CAD build for the part. Positions are in the model's coordinates, mm. A direction names the side the tool comes from. Round coordinates to 2 decimals unless told otherwise and drop trailing zeros. Loops run counter-clockwise (first coordinate to the right, second up) from the corner with the lowest first, then second, coordinate; pieces in that order, holes last. Notation, with made-up numbers: (11, -39) - (64, -39) arc R17 cw to (64, -35) - close; hole circle Ø3 at (19, 0). An arc over 180 degrees is marked (long way). Use one line per item in the form item = value.
Autodesk Inventor part; units mm, degrees
ref_plane "YZ Plane" through (0, 0, 0) normal (1, 0, 0) x (0, 1, 0)
ref_plane "XZ Plane" through (0, 0, 0) normal (0, 1, 0) x (-1, 0, 0)
ref_plane "XY Plane" through (0, 0, 0) normal (0, 0, 1) x (1, 0, 0)
sketch "Sketch1" plane through (0, 0, 0) normal (0, 0, 1) x (1, 0, 0)
  circle A0 centre (0, 0) radius 2.5
  dimension "d0" = 5
extrude "Extrusion1" add sketch "Sketch1" along normal blind 10
sketch "Sketch2" plane through (0, 0, 10) normal (0, 0, 1) x (1, 0, 0)
  circle A0 centre (0, 0) radius 3.5
  dimension "d3" = 7
extrude "Extrusion2" add sketch "Sketch2" along normal blind 4.5
sketch "Sketch3" plane through (0, 0, 14.5) normal (0, 0, 1) x (1, 0, 0)
  line L0 (-1.25, 1.55) -> (1.25, 1.55)
  line L1 (1.25, 1.55) -> (1.25, -1.55)
  line L2 (1.25, -1.55) -> (-1.25, -1.55)
  line L3 (-1.25, -1.55) -> (-1.25, 1.55)
  point P0 (0, 0)
  point P1 (-1.25, 0)
  point P2 (0, 1.55)
  dimension "d6" = 2.5
  dimension "d7" = 3.1
extrude "Extrusion3" cut sketch "Sketch3" against normal blind 4
sketch "Sketch4" plane through (0, 0, 0) normal (0, 0, -1) x (-1, 0, 0)
  circle A0 centre (0, 0) radius 0.5
  line L0 (2.5, -0.1) -> (-2.5, -0.1)
  line L1 (-2.5, -0.1) -> (-2.5, 0.1)
  line L2 (-2.5, 0.1) -> (2.5, 0.1)
  line L3 (2.5, 0.1) -> (2.5, -0.1)
  point P0 (0, -0.1)
  point P1 (2.5, 0)
  point P2 (-0.4899, 0.1)
  point P3 (-0.4899, -0.1)
  point P4 (0.4899, -0.1)
  point P5 (0.4899, 0.1)
  dimension "d10" = 1
  dimension "d11" = 5
  dimension "d12" = 0.2
extrude "Extrusion4" cut sketch "Sketch4" against normal blind 8
properties part number "Magnethalter"
1) Tool access for faces 4 (the flat face through (0, 1, 0)), 5 (the flat face through (1, -0.1, 4)), 6 (the flat face through (2, 0, 14.5)), 7 (the flat face through (1.25, 0, 13)), 8 (the flat face through (0, 0, 8)): list every direction of +Z, -Z, +X, -X, +Y, -Y with a clear straight run to the whole face (end or side of a thin tool).
Report:
face_4 = -Z, +X, -X, +Y, -Y
face_5 = -Z, +X, -X
face_6 = +Z, +X, -X, +Y, -Y
face_7 = +Z
face_8 = -Z
2) Slice it at A-A (x = 0). Write the cut outline in (y, z).
Report:
outline = (-3.5, 10) - (-2.5, 10) - (-2.5, 0) - (-0.5, 0) - (-0.5, 8) - (0.5, 8) - (0.5, 0) - (2.5, 0) - (2.5, 10) - (3.5, 10) - (3.5, 14.5) - (1.55, 14.5) - (1.55, 10.5) - (-1.55, 10.5) - (-1.55, 14.5) - (-3.5, 14.5) - close
3) Two-plate mould, pull along X, no slides. Class faces 1 (the cylindrical face through (3.233, 1.341, 12.218)), 2 (the flat face through (-1.25, 0, 13)), 3 (the flat face through (2, -2, 10)): +X half, -X half, draft (parallel to the pull), parting line (faces both ways), or undercut.
Report:
face_1 = parting line
face_2 = undercut
face_3 = draft
4) Slice it at D-D (z = 9). Write the cut outline in (x, y), plus the area to 3 significant figures.
Report:
outline = circle Ø5 at (0, 0)
area = 19.6 mm^2
5) Slice it at B-B (z = 13.25). Write the cut outline in (x, y), plus the area to 3 significant figures.
Report:
outline = circle Ø7 at (0, 0); hole (-1.25, -1.55) - (1.25, -1.55) - (1.25, 1.55) - (-1.25, 1.55) - close
area = 30.7 mm^2
6) Drill centre lines: probe 1 along Z at (x, y) = (-1.25, -2.75); probe 2 along Y at (x, z) = (-0.25, 4.25); probe 3 along Y at (x, z) = (-1.25, 3). Where is each one in solid material? Low to high.
Report:
probe_1 = 10 to 14.5
probe_2 = -2.49 to -0.43, 0.43 to 2.49
probe_3 = -2.17 to -0.1, 0.1 to 2.17
7) Slice it at C-C (y = 1). Write the cut outline in (x, z).
Report:
outline = (-3.35, 10) - (-2.29, 10) - (-2.29, 0) - (2.29, 0) - (2.29, 10) - (3.35, 10) - (3.35, 14.5) - (1.25, 14.5) - (1.25, 10.5) - (-1.25, 10.5) - (-1.25, 14.5) - (-3.35, 14.5) - close
8) Flat gauge pins, fed straight in: pin 1 (2 mm diameter, centred on x = -2.5, z = 11.5, fed in from -Y); pin 2 (0.8 mm diameter, centred on x = -0.5, z = 12.5, fed in from -Y); pin 3 (1 mm diameter, centred on y = 0, z = 4.5, fed in from -X); pin 4 (3 mm diameter, centred on x = 1, z = 5, fed in from -Y). Where does each tip first touch, or does it go through?
Report:
pin_1 = -3.16
pin_2 = -3.5
pin_3 = -2.5
pin_4 = -2.5
